Build history of the part. All positions in model axes, mm. A direction names the side the tool comes from. Round coordinates to 2 decimals unless told otherwise and drop trailing zeros. Write each loop counter-clockwise with the first axis right and the second up, starting at its lowest first coordinate (ties: lowest second). Pieces come first, ordered by that corner, then holes. Notation, with made-up numbers: (79.5, 33.25) -> (97.5, 33.25) arc R17 ccw to (97.5, 65.25) -> close; hole circle Ø2 at (-18.5, 41.25). An arc over 180 degrees is marked (long way). Answer in a Markdown table with one row per item.
```python
from build123d import *

# Parameters (mm, degrees)
F0_W      = 80
F0_H      = 40
F1_DEPTH  = 10
F2_W      = 10
F2_H      = 40
F3_DEPTH  = 30
F4_W      = 15
F4_H      = 40
F5_DEPTH  = 10
F7_DEPTH  = 40.001
F9_DEPTH  = 80.001
F10_R     = 7.5
F11_DEPTH = 20.001


with BuildPart() as f1:
    # F0 (on Top) → F1 (new body)
    with BuildSketch(Plane.XY):
        Rectangle(F0_W, F0_H)
    extrude(amount=F1_DEPTH)

    # F2 (on face) → F3 (join)
    with BuildSketch(Plane.XY.offset(10)):
        with Locations((-35, 0)):
            Rectangle(F2_W, F2_H)
    extrude(amount=F3_DEPTH)

    # F4 (on face) → F5 (join)
    with BuildSketch(Plane(origin=(0, 0, 0), x_dir=(1, 0, 0), z_dir=(0, 0, -1))):
        with Locations((32.5, 0)):
            Rectangle(F4_W, F4_H)
    extrude(amount=F5_DEPTH)

    # F6 (on face) → F7 (cut, through all)
    with BuildSketch(Plane.XZ.offset(20)):
        Polygon((40, 0), (35, -10), (40, -10), align=None)
    extrude(amount=-F7_DEPTH, mode=Mode.SUBTRACT)

    # F8 (on face) → F9 (cut, through all)
    with BuildSketch(Plane(origin=(-40, 0, 0), x_dir=(0, -1, 0), z_dir=(-1, 0, 0))):
        Polygon((5, 40), (-5, 40), (-5, 30), (-10, 30), (-10, 20), (10, 20), (10, 30), (5, 30), align=None)
    extrude(amount=-F9_DEPTH, mode=Mode.SUBTRACT)

    # F10 (on face) → F11 (cut, through all)
    with BuildSketch(Plane.XY.offset(10)):
        with Locations((5, 0)):
            Circle(F10_R)
    extrude(amount=-F11_DEPTH, mode=Mode.SUBTRACT)


solid = f1.part
```
Q1. Saw through at D-D on z = 1. Write the cut outline in (x, y).
A:
| item | result |
|---|---|
| outline | (-40, -20) -> (40, -20) -> (40, 20) -> (-40, 20) -> close; hole circle Ø15 at (5, 0) |
Q2. Wall check: line 1 (Z direction, x = -30.5, y = -5.5); line 2 (Y direction, x = 5, z = 4.75); line 3 (Z direction, x = 13, y = 9). Give the ranges that are in metal, low to high. Write a range as [from, to].
A:
| item | result |
|---|---|
| line 1 | [0, 20], [30, 40] |
| line 2 | [-20, -7.5], [7.5, 20] |
| line 3 | [0, 10] |
Q3. Two-plate mould, pull along Z, no slides. Class faces 1 (the cylindrical face through (11.93, -2.87, 5.07)), 2 (the flat face through (-35, -10, 25)), 3 (the flat face through (-35, 10, 25)), 4 (the flat face through (-35, 13, 40)): released by +Z, released by -Z, zero draft, split by the parting line, or undercut.
A:
| item | result |
|---|---|
| face 1 | zero draft |
| face 2 | undercut |
| face 3 | undercut |
| face 4 | released by +Z |
Q4. Which spindle directions (+Z, -Z, +X, -X, +Y, -Y) get a long thin tool onto all of the face, cutting with end or side? Do faces 5 (the flat face through (-30, 0, 18)), 6 (the flat face through (-35, -8, 30)), 7 (the flat face through (-8, 0, 0)), 8 (the flat face through (-35, -5, 35)). Say none if no direction does.
A:
| item | result |
|---|---|
| face 5 | +Z, +X, +Y, -Y |
| face 6 | +X, -X |
| face 7 | -Z, -X, +Y, -Y |
| face 8 | +Z, +X, -X |
Q5. Saw through at B-B on x = 5. Write the cut outline in (y, z), plus the area to 3 significant figures.
A:
| item | result |
|---|---|
| outline | (-20, 0) -> (-7.5, 0) -> (-7.5, 10) -> (-20, 10) -> close; (7.5, 0) -> (20, 0) -> (20, 10) -> (7.5, 10) -> close |
| area | 250 mm² |
Q6. Drop flat-ended pins along their axis: P1, Ø19.5, axis at x = 5, y = 0, coming from the -Z side; P2, Ø11, axis at x = -37, y = -3.5, coming from the +Z side; P3, Ø20, axis at x = 9.5, y = -3.5, coming from the +Z side; P4, Ø5, axis at y = -10, z = -5, coming from the -X side. Give the stop position or say it passes through.
A:
| item | result |
|---|---|
| P1 | z = 0 |
| P2 | z = 40 |
| P3 | z = 10 |
| P4 | x = 25 |
Q7. Saw through at A-A on z = 29. Write the cut outline in (x, y), plus the area to 3 significant figures.
A:
| item | result |
|---|---|
| outline | (-40, -20) -> (-30, -20) -> (-30, -10) -> (-40, -10) -> close; (-40, 10) -> (-30, 10) -> (-30, 20) -> (-40, 20) -> close |
| area | 200 mm² |
Q8. Saw through at C-C on y = 0. Write the cut outline in (x, z), plus the area to 3 significant figures.
A:
| item | result |
|---|---|
| outline | (-40, 0) -> (-2.5, 0) -> (-2.5, 10) -> (-30, 10) -> (-30, 20) -> (-40, 20) -> close; (12.5, 0) -> (25, 0) -> (25, -10) -> (35, -10) -> (40, 0) -> (40, 10) -> (12.5, 10) -> close |
| area | 875 mm² |
